Read the model definition and answer for the solid it produces. Units are mm, in the model's axes. Face numbers are marked on the shaded views. A direction names the side the tool comes from. Coordinates: 2 decimals unless noted, no trailing zeros. Order: outer loops, then holes, each group sorted by start corner. A loop starts at its lowest first (then second) coordinate and runs counter-clockwise, first axis right, second up. Notation, with made-up numbers: (53.25, -35) -> (104.25, -35) arc R29 ccw to (104.25, 3) -> close; hole circle Ø4 at (-10.75, -6). An arc over 180 degrees is marked (long way). Use CSV: the item, a comma, the result in double quotes.
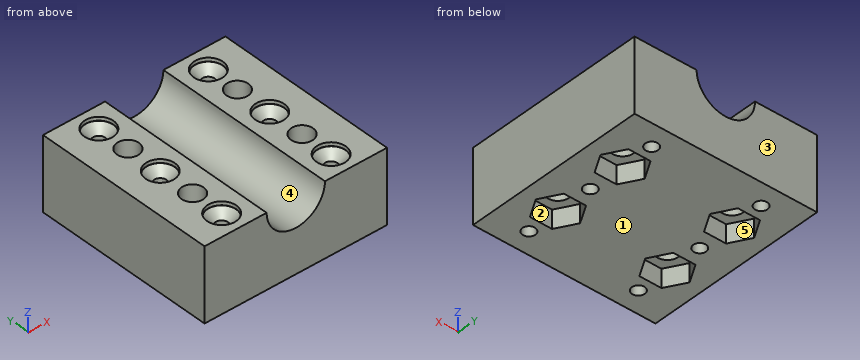
```python
from build123d import *

# Parameters (mm, degrees)
SKETCH1_W           = 50
SKETCH1_H           = 50
BOSS_EXTRUDE1_DEPTH = 20
SKETCH2_R           = 8
CUT_EXTRUDE1_DEPTH  = 67.942210384
SKETCH3_R           = 3
CUT_EXTRUDE2_DEPTH  = 43
CUT_EXTRUDE5_DEPTH  = 5
SKETCH7_R           = 1.75
CUT_EXTRUDE6_DEPTH  = 41
SKETCH9_R           = 4
CUT_EXTRUDE7_DEPTH  = 1
CHAMFER1_SIZE       = 2.2


with BuildPart() as part:
    # Sketch1 → Boss-Extrude1 (new body)
    with BuildSketch(Plane.XY):
        with Locations((25, 25)):
            Rectangle(SKETCH1_W, SKETCH1_H)
    extrude(amount=BOSS_EXTRUDE1_DEPTH)

    # Sketch2 → Cut-Extrude1 (cut)
    with BuildSketch(Plane(origin=(0, 50, 0), x_dir=(1, 0, 0), z_dir=(0, 1, 0))):
        with Locations((25, -20)):
            Circle(SKETCH2_R)
    extrude(amount=-CUT_EXTRUDE1_DEPTH, mode=Mode.SUBTRACT)

    # Sketch3 → Cut-Extrude2 (cut)
    with BuildSketch(Plane.XY.offset(20)):
        with Locations((10, 35)):
            Circle(SKETCH3_R)
        with Locations((10, 15)):
            Circle(SKETCH3_R)
        with Locations((40, 35)):
            Circle(SKETCH3_R)
        with Locations((40, 15)):
            Circle(SKETCH3_R)
    extrude(amount=-CUT_EXTRUDE2_DEPTH, mode=Mode.SUBTRACT)

    # Sketch6 → Cut-Extrude5 (cut)
    with BuildSketch(Plane(origin=(0, 0, 0), x_dir=(-1, 0, 0), z_dir=(0, 0, -1))):
        Polygon((-3.937822174, 15), (-6.968911087, 20.25), (-13.031088913, 20.25), (-16.062177826, 15), (-13.031088913, 9.75), (-6.968911087, 9.75), align=None)
        Polygon((-43.031088913, 20.25), (-46.062177826, 15), (-43.031088913, 9.75), (-36.968911087, 9.75), (-33.937822174, 15), (-36.968911087, 20.25), align=None)
        Polygon((-36.968911087, 29.75), (-33.937822174, 35), (-36.968911087, 40.25), (-43.031088913, 40.25), (-46.062177826, 35), (-43.031088913, 29.75), align=None)
        Polygon((-6.968911087, 29.75), (-3.937822174, 35), (-6.968911087, 40.25), (-13.031088913, 40.25), (-16.062177826, 35), (-13.031088913, 29.75), align=None)
    extrude(amount=-CUT_EXTRUDE5_DEPTH, mode=Mode.SUBTRACT)

    # Sketch7 → Cut-Extrude6 (cut)
    with BuildSketch(Plane.XY.offset(20)):
        with Locations((10, 6)):
            Circle(SKETCH7_R)
        with Locations((10, 25)):
            Circle(SKETCH7_R)
        with Locations((10, 44)):
            Circle(SKETCH7_R)
        with Locations((40, 44)):
            Circle(SKETCH7_R)
        with Locations((40, 25)):
            Circle(SKETCH7_R)
        with Locations((40, 6)):
            Circle(SKETCH7_R)
    extrude(amount=-CUT_EXTRUDE6_DEPTH, mode=Mode.SUBTRACT)

    # Sketch9 → Cut-Extrude7 (cut)
    with BuildSketch(Plane.XY.offset(20)):
        with Locations((10, 44)):
            Circle(SKETCH9_R)
        with Locations((10, 25)):
            Circle(SKETCH9_R)
        with Locations((10, 6)):
            Circle(SKETCH9_R)
        with Locations((40, 6)):
            Circle(SKETCH9_R)
        with Locations((40, 25)):
            Circle(SKETCH9_R)
        with Locations((40, 44)):
            Circle(SKETCH9_R)
    extrude(amount=-CUT_EXTRUDE7_DEPTH, mode=Mode.SUBTRACT)

    # Chamfer1
    chamfer1_edges = [part.edges().sort_by_distance(p)[0] for p in [
        (8.25, 44, 19),
        (8.25, 25, 19),
        (8.25, 6, 19),
        (38.25, 6, 19),
        (38.25, 25, 19),
        (38.25, 44, 19),
    ]]
    chamfer(chamfer1_edges, length=CHAMFER1_SIZE)


solid = part.part
```
Item 1: Find section A-A, the plane z = 9.5. Give the number of separate pieces and of enclosed holes in the cut face, then the cut area to 3 significant figures.
Return value:
separate pieces,"1"
enclosed holes,"10"
area,"2,330 mm^2"
Item 2: Straight lines are drawn through the part: line 1 along X through (y, z) = (25.5, 4.25); line 2 along X through (y, z) = (16, 6.5); line 3 along Y through (x, z) = (41.5, 1). For each, find the intervals that lie inside material, in ascending order.
Return value:
line 1,"x = 0 to 8.32, 11.68 to 38.32, 41.68 to 50"
line 2,"x = 0 to 7.17, 12.83 to 37.17, 42.83 to 50"
line 3,"y = 0 to 5.1, 6.9 to 9.75, 20.25 to 24.1, 25.9 to 29.75, 40.25 to 43.1, 44.9 to 50"
Item 3: The mould has two halves that part along Y. Classify the marked faces 1, 2 and 3: +Y half, -Y half, draft (parallel to the pull), parting line (faces both ways), or undercut.
Return value:
face 1,"draft"
face 2,"undercut"
face 3,"+Y half"
Item 4: Find section B-B, the plane y = 6. Give the vertices of the cut face in (x, z), then the cut area to 3 significant figures.
Return value:
outline,"(0, 0) -> (8.25, 0) -> (8.25, 16.8) -> (6.05, 19) -> (6, 19) -> (6, 20) -> (0, 20) -> close; (11.75, 0) -> (38.25, 0) -> (38.25, 16.8) -> (36.05, 19) -> (36, 19) -> (36, 20) -> (33, 20) arc R8 cw to (17, 20) -> (14, 20) -> (14, 19) -> (13.95, 19) -> (11.75, 16.8) -> close; (41.75, 0) -> (50, 0) -> (50, 20) -> (44, 20) -> (44, 19) -> (43.95, 19) -> (41.75, 16.8) -> close"
area,"741 mm^2"
Item 5: A tool of negligible diameter and unlimited length cuts with its end or side. For the marked faces 4 and 5, from which of +Z, -Z, +X, -X, +Y, -Y can it reach the whole face along a straight path? Write none if from no direction.
Return value:
face 4,"+Z, +Y, -Y"
face 5,"-Z"
Item 6: Each of these flat-tipped pins is pushed along its axis until it touches: P1, Ø4, axis at x = 9.5, y = 25, coming from the +Z side; P2, Ø5.5, axis at x = 40, y = 44, coming from the +Z side; P3, Ø2.5, axis at x = 9, y = 43.5, coming from the +Z side. Where does it stop, or does it pass through?
Return value:
P1,"stops at z = 17.55"
P2,"stops at z = 17.8"
P3,"stops at z = 17.42"
Item 7: Find section D-D, the plane x = 35. Give the vertices of the cut face in (y, z), then the cut area to 3 significant figures.
Return value:
outline,"(0, 0) -> (13.16, 0) -> (13.16, 5) -> (16.84, 5) -> (16.84, 0) -> (33.16, 0) -> (33.16, 5) -> (36.84, 5) -> (36.84, 0) -> (50, 0) -> (50, 20) -> (0, 20) -> close"
area,"963 mm^2"
